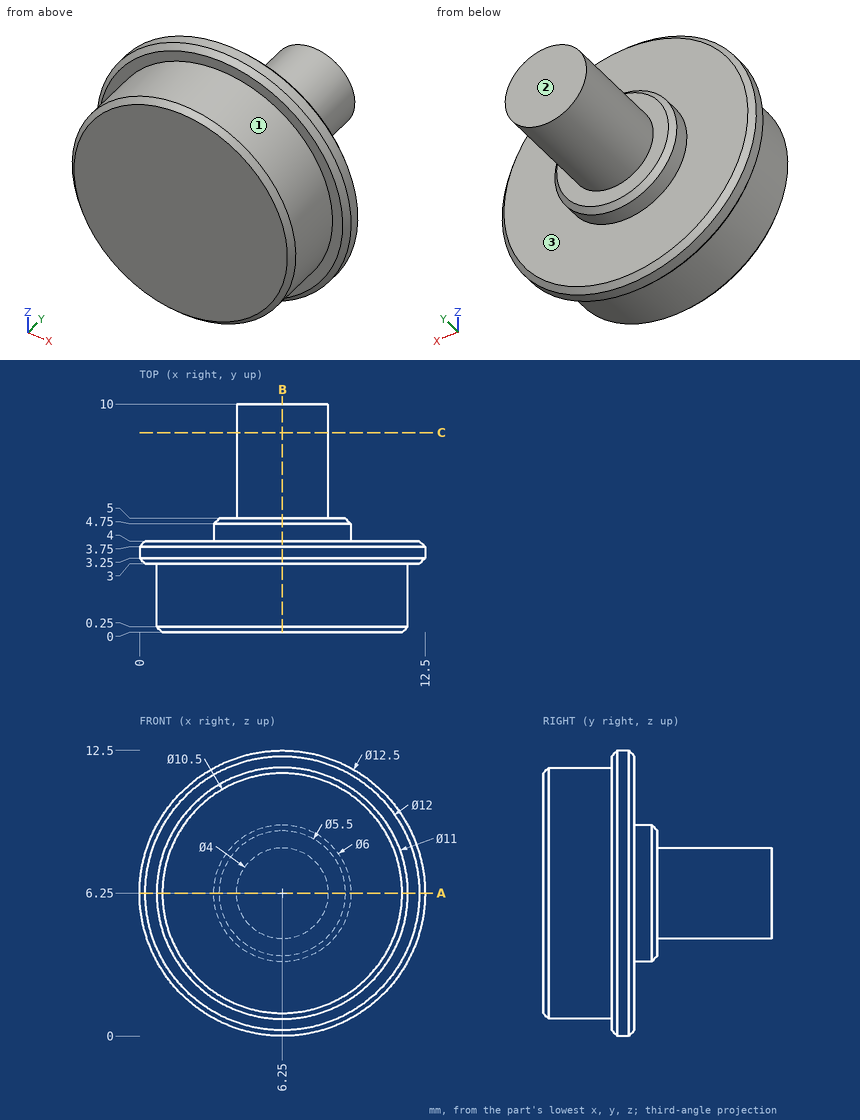
For this review, use the dimensioned drawing (mm, ordinates from the lowest corner) and the shaded views. A direction names the side the tool comes from. Give positions to 0.01 mm unless a question says otherwise; leave off trailing zeros. Order: outer loops, then holes, each group sorted by start corner. A loop starts at its lowest first (then second) coordinate and runs counter-clockwise, first axis right, second up.
1) Take a section at C-C (y = 8.75). Give the boundary of the cut face in (x, z), then the cut area to 3 significant figures.
2) Insertion check: pin 1 (5 mm diameter, centred on x = 6.5, y = 8.5, fed in from +Z); pin 2 (6 mm diameter, centred on x = 9, z = 6, fed in from -Y); pin 3 (5 mm diameter, centred on x = 11, y = 4.5, fed in from -Z); pin 4 (5 mm diameter, centred on x = 3.5, y = 4, fed in from +Z). Each pin has a flat end and moves straight along its axis. Give the tip position at first contact, or say it passes through.
3) Wall thickness on line 1 (Y direction, x = 2.75, z = 8.75); line 2 (Y direction, x = 7.25, z = 1); line 3 (X direction, y = 5.25, z = 6): over which ranges is each line inside the solid? List them lowest first.
4) For the marked faces 1, 2 and 3, list the 3-axis set-ups (+Z, -Z, +X, -X, +Y, -Y) from which the entire face can be reached by the end or side of a thin tool; tool diameter is ignored.
5) Take a section at B-B (x = 6.25). Give the boundary of the cut face in (y, z).
6) Take a section at A-A (z = 6.25). Give the boundary of the cut face in (x, y).
Derived:
1. outline: circle Ø4 at (6.25, 6.25)
1. area: 12.6 mm2
2. pin 1: stops at z = 8.25
2. pin 2: stops at y = 0
2. pin 3: stops at z = 0.46
2. pin 4: stops at z = 12.49
3. line 1: y = 0 to 4
3. line 2: y = 0.09 to 4
3. line 3: x = 4.27 to 8.23
4. face 1: -Y
4. face 2: +Z, -Z, +X, -X, +Y
4. face 3: +Y
5. outline: (0, 1) - (0.25, 0.75) - (3, 0.75) - (3, 0.25) - (3.25, 0) - (3.75, 0) - (4, 0.25) - (4, 3.25) - (4.75, 3.25) - (5, 3.5) - (5, 4.25) - (10, 4.25) - (10, 8.25) - (5, 8.25) - (5, 9) - (4.75, 9.25) - (4, 9.25) - (4, 12.25) - (3.75, 12.5) - (3.25, 12.5) - (3, 12.25) - (3, 11.75) - (0.25, 11.75) - (0, 11.5) - close
6. outline: (0, 3.25) - (0.25, 3) - (0.75, 3) - (0.75, 0.25) - (1, 0) - (11.5, 0) - (11.75, 0.25) - (11.75, 3) - (12.25, 3) - (12.5, 3.25) - (12.5, 3.75) - (12.25, 4) - (9.25, 4) - (9.25, 4.75) - (9, 5) - (8.25, 5) - (8.25, 10) - (4.25, 10) - (4.25, 5) - (3.5, 5) - (3.25, 4.75) - (3.25, 4) - (0.25, 4) - (0, 3.75) - close
